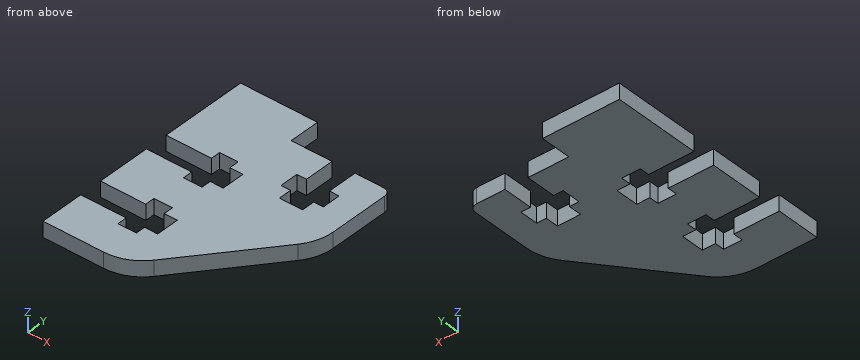
```python
from build123d import *

# Parameters (mm, degrees)
BOSS_EXTRUDE1_DEPTH = 2


with BuildPart() as part:
    # Model → Boss-Extrude1 (new body)
    with BuildSketch(Plane.XY):
        with BuildLine():
            Line((10, 5.75), (8.3, 5.75))
            Line((8.3, 5.75), (8.3, 4.5))
            Line((8.3, 4.5), (5.9, 4.5))
            Line((5.9, 4.5), (5.9, 5.75))
            Line((5.9, 5.75), (0, 5.75))
            Line((0, 5.75), (0, 0))
            Line((0, 0), (7.88848997, 0))
            ThreePointArc((7.88848997, 0), (10.472480827, 0.584929248), (12.552654408, 2.225669584))
            Line((12.552654408, 2.225669584), (21.664164438, 13.485304109))
            ThreePointArc((21.664164438, 13.485304109), (22.656190707, 15.257758734), (23, 17.259634525))
            Line((23, 17.259634525), (23, 25.1))
            ThreePointArc((23, 25.1), (22.707106781, 25.807106781), (22, 26.1))
            Line((22, 26.1), (18.306018336, 26.1))
            Line((18.306018336, 26.1), (18.306018336, 22.2))
            Line((18.306018336, 22.2), (19.556018336, 22.2))
            Line((19.556018336, 22.2), (19.556018336, 19.8))
            Line((19.556018336, 19.8), (18.306018336, 19.8))
            Line((18.306018336, 19.8), (18.306018336, 18.1))
            Line((18.306018336, 18.1), (15.306018336, 18.1))
            Line((15.306018336, 18.1), (15.306018336, 19.8))
            Line((15.306018336, 19.8), (14.056018336, 19.8))
            Line((14.056018336, 19.8), (14.056018336, 22.2))
            Line((14.056018336, 22.2), (15.306018336, 22.2))
            Line((15.306018336, 22.2), (15.306018336, 26.1))
            Line((15.306018336, 26.1), (10, 26.1))
            Line((10, 26.1), (10, 30.1))
            Line((10, 30.1), (0, 30.1))
            Line((0, 30.1), (0, 18.75))
            Line((0, 18.75), (5.9, 18.75))
            Line((5.9, 18.75), (5.9, 20))
            Line((5.9, 20), (8.3, 20))
            Line((8.3, 20), (8.3, 18.75))
            Line((8.3, 18.75), (10, 18.75))
            Line((10, 18.75), (10, 15.75))
            Line((10, 15.75), (8.3, 15.75))
            Line((8.3, 15.75), (8.3, 14.5))
            Line((8.3, 14.5), (5.9, 14.5))
            Line((5.9, 14.5), (5.9, 15.75))
            Line((5.9, 15.75), (0, 15.75))
            Line((0, 15.75), (0, 8.75))
            Line((0, 8.75), (5.9, 8.75))
            Line((5.9, 8.75), (5.9, 10))
            Line((5.9, 10), (8.3, 10))
            Line((8.3, 10), (8.3, 8.75))
            Line((8.3, 8.75), (10, 8.75))
            Line((10, 8.75), (10, 5.75))
        make_face()
    extrude(amount=BOSS_EXTRUDE1_DEPTH)


solid = part.part
```
Geometry: final body of the model. Coordinates: model frame, mm. Round coordinates to 2 decimals unless told otherwise and drop trailing zeros. Order: outer loops, then holes, each group sorted by start corner. A loop starts at its lowest first (then second) coordinate and runs counter-clockwise, first axis right, second up. Notation, with made-up numbers: (-7, 54.25) - (-2, 54.25) arc R21 ccw to (-2, 59.25) - close; hole circle Ø5 at (-28.5, 15.25). An arc over 180 degrees is marked (long way). Write item = value, one per line. Start each with the question number.
Q1. Cut plane B-B on x = 6.5. Return the cut outline in (y, z).
Q2. Pin query (flat end, axial travel): pin 1 (1 mm diameter, centred on x = 20.5, z = 1, fed in from +Y); pin 2 (0.8 mm diameter, centred on x = 9.5, z = 1, fed in from -Y); pin 3 (0.6 mm diameter, centred on x = 15, z = 1, fed in from -Y). Return the tip coordinate at first contact, or that it passes through.
Q3. Ray query, line 1 (Y direction, x = 3, z = 0.4); line 2 (Y direction, x = 6.75, z = 0.75); line 3 (X direction, y = 20.5, z = 0.2). Return the intervals inside material, ascending. Write a range as from..to.
Q4. Cut plane C-C on y = 7.5. Return the cut outline in (x, z), and give its area (3 significant figures).
Q5. Cut plane D-D on x = 13.5. Return the cut outline in (y, z), and give its area (3 significant figures).
Q6. Cut plane A-A on y = 21.5. Return the cut outline in (x, z).
Outcome:
q1.outline = (0, 0) - (4.5, 0) - (4.5, 2) - (0, 2) - close; (10, 0) - (14.5, 0) - (14.5, 2) - (10, 2) - close; (20, 0) - (30.1, 0) - (30.1, 2) - (20, 2) - close
q2.pin_1 = 26.1
q2.pin_2 = 0.12
q2.pin_3 = 4.88
q3.line_1 = 0..5.75, 8.75..15.75, 18.75..30.1
q3.line_2 = 0..4.5, 10..14.5, 20..30.1
q3.line_3 = 0..14.06, 19.56..23
q4.outline = (10, 0) - (16.82, 0) - (16.82, 2) - (10, 2) - close
q4.area = 13.6 mm^2
q5.outline = (3.4, 0) - (26.1, 0) - (26.1, 2) - (3.4, 2) - close
q5.area = 45.4 mm^2
q6.outline = (0, 0) - (14.06, 0) - (14.06, 2) - (0, 2) - close; (19.56, 0) - (23, 0) - (23, 2) - (19.56, 2) - close
